from build123d import *

# Parameters (mm, degrees)
SKETCH1_R           = 25.5
BOSS_EXTRUDE1_DEPTH = 128
FILLET2_R           = 5
SKETCH2_R           = 18.5
BOSS_EXTRUDE2_DEPTH = 4
FILLET5_R           = 15
SKETCH3_R           = 5
CUT_EXTRUDE1_DEPTH  = 137.83749488


# Read off the part's stored shape, not the designer's step: Shell1
with BuildPart() as part:
    # Sketch1 → Boss-Extrude1 (new body)
    with BuildSketch(Plane(origin=(0, 0, 0), x_dir=(1, 0, 0), z_dir=(0, 1, 0))):
        with Locations(Location((0, 0, 0), (0, 0, 270))):
            Circle(SKETCH1_R)
    extrude(amount=BOSS_EXTRUDE1_DEPTH)

    # Fillet2
    fillet2_edges = [part.edges().sort_by_distance(p)[0] for p in [
        (0, 128, -25.5),
    ]]
    fillet(fillet2_edges, radius=FILLET2_R)

    # Sketch2 → Boss-Extrude2 (add)
    with BuildSketch(Plane(origin=(0, 128, 0), x_dir=(1, 0, 0), z_dir=(0, 1, 0))):
        with Locations(Location((0, 0, 0), (0, 0, 270))):
            Circle(SKETCH2_R)
    extrude(amount=BOSS_EXTRUDE2_DEPTH)

    # Fillet5
    # the kernel refuses this fillet: 15 mm, written as the material it takes off along each edge
    with BuildSketch(Plane(origin=(0, 132, 0), x_dir=(0, 0, 1), z_dir=(-1, 0, 0))) as fillet5_piece_1:
        with BuildLine():
            CenterArc((8.301960973, -15), FILLET5_R, 47.166571934, 42.833428066)
            Line((8.301960973, 0), (8.301960973, 0.3))
            Line((8.301960973, 0.3), (18.5, 0.3))
            Line((18.5, 0.3), (18.8, 0))
            ThreePointArc((18.8, 0), (18.8, -2), (18.703960781, -3.78))
            Line((18.703960781, -3.78), (18.5, -4))
        make_face()
    revolve(axis=Axis((0, 132, 0), (0, 1, 0)), mode=Mode.SUBTRACT)

    # Shell1 outline → Shell1 (revolve, cut)
    with BuildSketch(Plane.XY):
        with BuildLine():
            Line((24, 0), (24, 123))
            ThreePointArc((24, 123), (22.974873734, 125.474873734), (20.5, 126.5))
            Line((20.5, 126.5), (17.893624019, 126.5))
            ThreePointArc((17.893624019, 126.5), (13.498113395, 129.459935794), (8.301960973, 130.5))
            Line((8.301960973, 130.5), (0, 130.5))
            Line((0, 130.5), (0, 0))
            Line((0, 0), (24, 0))
        make_face()
    revolve(axis=Axis((0, 0, 0), (0, 1, 0)), mode=Mode.SUBTRACT)

    # Sketch3 → Cut-Extrude1 (cut, through all)
    with BuildSketch(Plane(origin=(0, 132, 0), x_dir=(1, 0, 0), z_dir=(0, 1, 0))):
        with Locations(Location((0, 0, 0), (0, 0, 270))):
            Circle(SKETCH3_R)
    extrude(amount=-CUT_EXTRUDE1_DEPTH, mode=Mode.SUBTRACT)


solid = part.part
The listing builds one solid part. Answer for the finished solid, in the listing's coordinates (mm). A direction names the side the tool comes from. Coordinates: 2 decimals unless noted, no trailing zeros. Write each loop counter-clockwise with the first axis right and the second up, starting at its lowest first coordinate (ties: lowest second). Pieces come first, ordered by that corner, then holes. Notation, with made-up numbers: (7.5, -27) - (48.5, -27) arc R22 cw to (48.5, -17) - close; hole circle Ø8 at (87, -16.75). An arc over 180 degrees is marked (long way). Put each result on its own line as item: value.
1. The part is cut by section A-A on y = 66.5. Give the vertices of the cut face in (x, z), plus the area to 3 significant figures.
Answer sheet:
outline: circle Ø51 at (0, 0); hole circle Ø48 at (0, 0)
area: 233 mm^2
2. Determine the mould class of faces 4 (the face through (-19, 0, 15)), 5 (the face through (-24.9, 60.6, -5.5)), 6 (the face through (-4.88, 131.26, -1.08)) for opening direction Z: pulls with the +Z half, pulls with the -Z half, needs draft (parallel to the pull), parting line crosses it, or undercut.
Answer sheet:
face 4: needs draft
face 5: parting line crosses it
face 6: undercut
3. A tool of negligible diameter and unlimited length cuts with its end or side. For faces 1 (the face through (-4, 132, 4)), 2 (the face through (-23.977, 62.361, -1.055)), 3 (the face through (15.3, 128, -10.7)), from which of +Z, -Z, +X, -X, +Y, -Y can it reach the whole face along a straight path? Write none if from no direction.
Answer sheet:
face 1: +Z, -Z, +X, -X, +Y
face 2: -Y
face 3: +Y
4. Flat-ended cylindrical pins translate along their axes: pin 1 Ø6 at (y, z) = (94, 17.5) entering from -X; pin 2 Ø3 at (y, z) = (16.5, -5) entering from -X; pin 3 Ø8 at (x, y) = (1, 69.5) entering from -Z; pin 4 Ø10 at (x, z) = (2, -17.5) entering from -Y. Find the tip coordinate at first contact, or state that the pin passes through.
Answer sheet:
pin 1: stops at x = -20.98
pin 2: stops at x = -25.26
pin 3: stops at z = -25.5
pin 4: stops at y = 125.79
5. Find the intervals of material crossed by line 1 along Z through (x, y) = (0.5, 118); line 2 along X through (y, z) = (112, -13.5); line 3 along X through (y, z) = (73.5, 15) (3 decimals), in increasing order. Write a range as from..to.
Answer sheet:
line 1: z = -25.5..-23.99, 23.99..25.5
line 2: x = -21.63..-19.84, 19.84..21.63
line 3: x = -20.622..-18.735, 18.735..20.622
